Read the model definition and answer for the solid it produces. Units are mm, in the model's axes. Face numbers are marked on the shaded views. A direction names the side the tool comes from. Round coordinates to 2 decimals unless told otherwise and drop trailing zeros. Order: outer loops, then holes, each group sorted by start corner. A loop starts at its lowest first (then second) coordinate and runs counter-clockwise, first axis right, second up. Notation, with made-up numbers: (-9.5, 9.5) - (33.5, 9.5) arc R24 cw to (33.5, 35.5) - close; hole circle Ø10 at (-8.75, 68). An arc over 180 degrees is marked (long way). Answer as a JSON object with one key per item and string values. Group by question number.
Q1. Given pin 1 Ø2.5 at (y, z) = (0, 12.7) entering from -X; pin 2 Ø5 at (x, z) = (33, -8.5) entering from +Y; pin 3 Ø1.5 at (x, y) = (-5.5, 31) entering from -Z; pin 4 Ø12 at (x, y) = (27.5, -6) entering from +Z, each flat-ended and moving along its own axis, determine where each tip first touches the part or whether it passes through.
Q2. A tool of negligible diameter and unlimited length cuts with its end or side. For the marked faces 5, 6 and 7, from which of +Z, -Z, +X, -X, +Y, -Y can it reach the whole face along a straight path? Write none if from no direction.
Q3. A cutting plane is placed at C-C on x = 8.5. Determine the outline of the cut face in (y, z).
Q4. Consider line 1 (X direction, y = 26, z = 52.5); line 2 (Z direction, x = 62, y = 0). Determine where each line is inside the solid, lowest interval first.
Q5. A cutting plane is placed at A-A on z = 30. Determine the outline of the cut face in (x, y).
Q6. The mould has two halves that part along X. Classify the marked faces 1, 2, 3 and 4: pulls with the +X half, pulls with the -X half, needs draft (parallel to the pull), parting line crosses it, or undercut.
Q7. A cutting plane is placed at B-B on y = -29. Determine the outline of the cut face in (x, z).
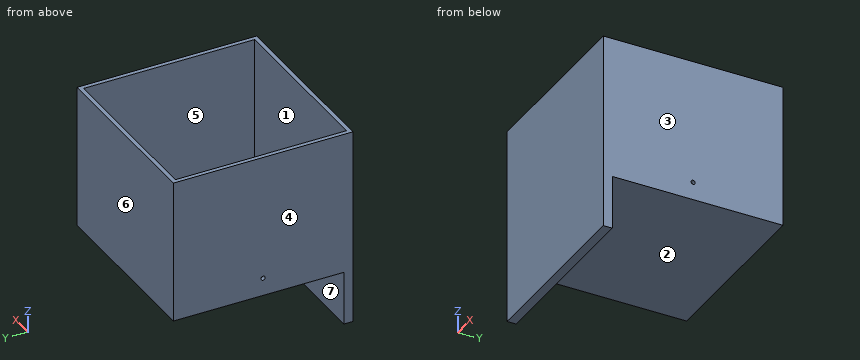
```python
from build123d import *

# Parameters (mm, degrees)
F0_W     = 127
F0_H     = 127
F1_DEPTH = 101.6
F2_T     = -3
F4_W     = 127
F4_H     = 38.1
F5_DEPTH = 6.35
F6_D     = 3


with BuildPart() as f1:
    # F0 (on Top) → F1 (new body)
    with BuildSketch(Plane.XY):
        Rectangle(F0_W, F0_H)
    extrude(amount=F1_DEPTH)

    # F2
    f2_openings = [f1.faces().sort_by_distance(p)[0] for p in [
        (0, 0, 101.6),
    ]]
    offset(amount=F2_T, openings=f2_openings)

    # F4 (on face) → F5 (join)
    with BuildSketch(Plane.XZ.offset(63.5)):
        with Locations((0, -19.05)):
            Rectangle(F4_W, F4_H)
    extrude(amount=-F5_DEPTH)

    # F6 (through all)
    with Locations(Plane.YZ.offset(63.5)):
        with Locations((0, 12.7)):
            Hole(F6_D / 2)


solid = f1.part
```
Result set:
{
 "1": {"pin 1": "passes through", "pin 2": "stops at y = -57.15", "pin 3": "stops at z = 0", "pin 4": "stops at z = 3"},
 "2": {"face 5": "+Z", "face 6": "+Z, -Z, +X, -X, +Y", "face 7": "-Z, +X, -X, +Y"},
 "3": {"outline": "(-63.5, -38.1) - (-57.15, -38.1) - (-57.15, 0) - (63.5, 0) - (63.5, 101.6) - (60.5, 101.6) - (60.5, 3) - (-60.5, 3) - (-60.5, 101.6) - (-63.5, 101.6) - close"},
 "4": {"line 1": "x = -63.5 to -60.5, 60.5 to 63.5", "line 2": "z = 0 to 11.2, 14.2 to 101.6"},
 "5": {"outline": "(-63.5, -63.5) - (63.5, -63.5) - (63.5, 63.5) - (-63.5, 63.5) - close; hole (-60.5, -60.5) - (60.5, -60.5) - (60.5, 60.5) - (-60.5, 60.5) - close"},
 "6": {"face 1": "undercut", "face 2": "needs draft", "face 3": "pulls with the +X half", "face 4": "pulls with the -X half"},
 "7": {"outline": "(-63.5, 0) - (63.5, 0) - (63.5, 101.6) - (60.5, 101.6) - (60.5, 3) - (-60.5, 3) - (-60.5, 101.6) - (-63.5, 101.6) - close"}
}
